Autodesk Inventor part; units mm, degrees
ref_plane "Start Plane" through (0, 0, 27.94) normal (0, 0, 1) x (1, 0, 0)
ref_plane "End Plane" through (0, 0, 472.44) normal (0, 0, 1) x (1, 0, 0)
ref_plane "Work Plane4" through (259.08, -25.4, 670.56) normal (-0.6, 0, 0.8) x (0.8, 0, 0.6)
ref_plane "Start Plane" through (0, 0, 27.94) normal (0, 0, 1) x (1, 0, 0)
ref_plane "End Plane" through (0, 0, 472.44) normal (0, 0, 1) x (1, 0, 0)
sketch "Sketch" plane through (0, 0, 0) normal (0, 0, 1) x (1, 0, 0)
  line L0 (-25.4, -25.4) -> (-25.4, 25.4)
  line L1 (-12.7, 38.1) -> (12.7, 38.1)
  line L2 (25.4, 25.4) -> (25.4, -25.4)
  line L3 (12.7, -38.1) -> (-12.7, -38.1)
  arc A0 (-25.4, -25.4) -> (-12.7, -38.1) centre (-12.7, -25.4) ccw
  arc A1 (-12.7, 38.1) -> (-25.4, 25.4) centre (-12.7, 25.4) ccw
  arc A2 (25.4, 25.4) -> (12.7, 38.1) centre (12.7, 25.4) ccw
  arc A3 (12.7, -38.1) -> (25.4, -25.4) centre (12.7, -25.4) ccw
  arc A4 (-12.7, 31.75) -> (-19.05, 25.4) centre (-12.7, 25.4) ccw
  line L4 (-12.7, 31.75) -> (12.7, 31.75)
  arc A5 (19.05, 25.4) -> (12.7, 31.75) centre (12.7, 25.4) ccw
  line L5 (19.05, 25.4) -> (19.05, -25.4)
  arc A6 (12.7, -31.75) -> (19.05, -25.4) centre (12.7, -25.4) ccw
  line L6 (12.7, -31.75) -> (-12.7, -31.75)
  arc A7 (-19.05, -25.4) -> (-12.7, -31.75) centre (-12.7, -25.4) ccw
  line L7 (-19.05, -25.4) -> (-19.05, 25.4)
  line L8 (0, 57.0224) -> (0, -57.0224) construction
  line L9 (-39.2424, 0) -> (39.2424, 0) construction
  dimension "d10" = 76.2
  dimension "d11" = 50.8
  dimension "d12" = 6.35
  dimension "d15" = 38.1
  dimension "d16" = 25.4
  dimension "d17" = 12.7
extrude "Body" add sketch "Sketch" along normal up to surface (444.5 mm away) from surface at 27.94
sketch "Sketch3" plane through (0, 0, 0) normal (0, 0, 1) x (1, 0, 0)
  line L0 (0, 0) -> (10, 0)
ref_plane "Work Plane3" through (0, 0, 0) normal (0, -1, 0) x (1, 0, 0)
ref_plane "Work Plane4" through (259.08, -25.4, 670.56) normal (-0.6, 0, 0.8) x (0.8, 0, 0.6)
split "Split1" plane through (259.08, -25.4, 670.56) removes the side toward (-0.6, 0, 0.8)
ref_plane "Work Plane5" through (-259.08, -25.4, -162.56) normal (0.6, 0, -0.8) x (-0.8, 0, -0.6)
split "Split2" plane through (-259.08, -25.4, -162.56) removes the side toward (0.6, 0, -0.8)
ref_plane "Work Plane6" through (223.52, -25.4, 167.64) normal (0.8, 0, 0.6) x (0.6, 0, -0.8)
split "Split3" plane through (223.52, -25.4, 167.64) removes the side toward (0.8, 0, 0.6)
ref_plane "Work Plane7" through (-480.568, -25.4, 166.624) normal (-0.28, 0, -0.96) x (-0.96, 0, 0.28)
split "Split4" plane through (-480.568, -25.4, 166.624) removes the side toward (-0.28, 0, -0.96)
sketch "Sketch4" plane through (0, 0, 0) normal (0, -1, 0) x (1, 0, 0)
  line L0 (-2, 27.94) -> (12, 27.94)
  line L1 (-2, 472.44) -> (12, 472.44)
  dimension "d19" = 444.5
equation "\"d10\" = G_H"
equation "\"d11\" = G_W"
equation "\"d12\" = G_T"
equation "\"d15\" = 0.5 * d10"
equation "\"d16\" = 0.5 * d11"
equation "\"d17\" = G_IR"
equation "\"d3\" = G_L"
equation "\"G_W\" = 50.8"
equation "\"G_H\" = 76.2"
equation "\"G_T\" = 6.35"
equation "\"G_IR\" = 12.7"
equation "\"G_L\" = d19"
equation "\"G_OFFSET_START\" = -27.94"
equation "\"G_OFFSET_END\" = -35.56"
equation "\"d13\" = -G_OFFSET_START"
equation "\"d14\" = G_OFFSET_END + B_L"
equation "\"B_L\" = 508"
properties part number "AISC - 3 x 2 x 1/4 - 17.5" material "Steel, Mild"
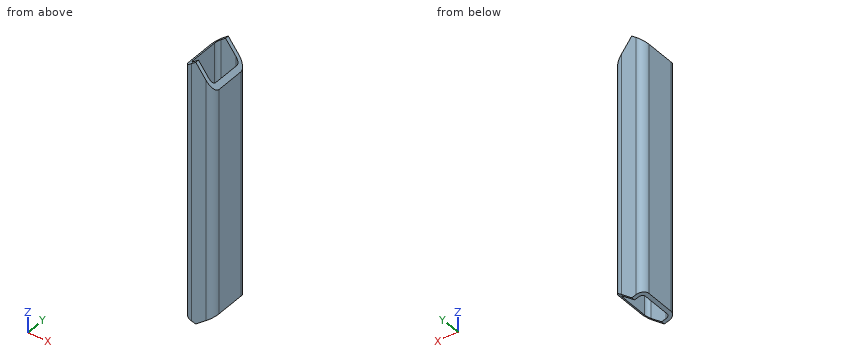
Here's how the part is built. I have some questions about the finished solid (model axes, mm). Round coordinates to 2 decimals unless told otherwise and drop trailing zeros. Write each loop counter-clockwise with the first axis right and the second up, starting at its lowest first coordinate (ties: lowest second). Pieces come first, ordered by that corner, then holes.
1. Suppose I cut it at B-B (x = 8). List the corners of the cut face in (y, z) for me, and give its area (3 significant figures).
2. Suppose I cut it at C-C (z = 82). List the corners of the cut face in (x, y) for me, and give its area (3 significant figures).
3. Will these pins go through, and if not, where does the flat tip stop? pin 1 Ø4 at (x, z) = (16, 408.5) entering from -Y; pin 2 Ø4 at (x, z) = (18.5, 135) entering from -Y; pin 3 Ø12 at (x, z) = (19.5, 99) entering from +Y.
4. Suppose I cut it at A-A (y = -17). List the corners of the cut face in (x, z) for me, and give its area (3 significant figures).
5. I need wall thicknesses on L1, parallel to Y at x = -5.5, z = 366; L2, parallel to X at y = -19, z = 421; L3, parallel to Y at x = -17, z = 55.5. Which ranges of each line are inside material? Lowest first, please.
Answer sheet:
1. outline: (-38.1, 37.75) - (-31.75, 37.75) - (-31.75, 455) - (-38.1, 455) - close; (31.75, 37.75) - (38.1, 37.75) - (38.1, 455) - (31.75, 455) - close
1. area: 5,300 mm2
2. outline: (-25.4, -25.4) arc R12.7 ccw to (-12.7, -38.1) - (12.7, -38.1) arc R12.7 ccw to (25.4, -25.4) - (25.4, 25.4) arc R12.7 ccw to (12.7, 38.1) - (-12.7, 38.1) arc R12.7 ccw to (-25.4, 25.4) - close; hole (-19.05, -25.4) arc R6.35 ccw to (-12.7, -31.75) - (12.7, -31.75) arc R6.35 ccw to (19.05, -25.4) - (19.05, 25.4) arc R6.35 ccw to (12.7, 31.75) - (-12.7, 31.75) arc R6.35 ccw to (-19.05, 25.4) - close
2. area: 1,350 mm2
3. pin 1: stops at y = -38.03
3. pin 2: stops at y = -37.52
3. pin 3: stops at y = 38.07
4. outline: (-25.4, 33.87) - (-19.05, 32.01) - (-19.05, 461.96) - (-25.4, 457.2) - close; (19.05, 46.04) - (25.4, 50.8) - (25.4, 431.8) - (19.05, 440.27) - close
4. area: 5,170 mm2
5. L1: y = -38.1 to -31.75, 31.75 to 38.1
5. L2: x = -25.4 to -19.05, 19.05 to 25.4
5. L3: y = -37.35 to -30.07, 30.07 to 37.35
